Part model, mm, in its own coordinate system. A direction names the side the tool comes from. Round coordinates to 2 decimals unless told otherwise and drop trailing zeros. Write each loop counter-clockwise with the first axis right and the second up, starting at its lowest first coordinate (ties: lowest second). Pieces come first, ordered by that corner, then holes. Notation, with made-up numbers: (-38.75, 86) -> (8.25, 86) arc R20 cw to (8.25, 115) -> close; hole circle Ø10 at (55.5, 48). An arc over 180 degrees is marked (long way). Return JSON: item names as keys, results as strings. Group by question number.
(1) Saw through at A-A (y = 6.25). List the corners of the cut face in (x, z).
(2) Mould opens along Z. For faces 3 (the flat face through (0, 12, 0)), 4 (the flat face through (0, 9.8, 0)), 5 (the cylindrical face through (0.66, 9.931, -14.985)), 6 (the cylindrical face through (-2.88, 5.59, 0.64)) say: +Z half, -Z half, draft (parallel to the pull), parting line (faces both ways), or undercut.
(3) Tool access for faces 1 (the cylindrical face through (0.66, 8.246, -14.985)), 2 (the cylindrical face through (-4.43, 8.75, 14.07)): list every direction of +Z, -Z, +X, -X, +Y, -Y with a clear straight run to the whole face (end or side of a thin tool).
(4) Drill centre lines: L1, parallel to X at y = 6.5, z = 0; L2, parallel to Y at x = -1.25, z = -0.5; L3, parallel to X at y = 5, z = 1.5. Where is each one in solid material? Low to high. Write a range as from..to.
(5) Drop flat-ended pins along their axis: pin 1 Ø1.5 at (y, z) = (9, -6.5) entering from -X; pin 2 Ø3 at (y, z) = (7.5, -2) entering from +X; pin 3 Ø1 at (x, z) = (7, 11) entering from +Y. Give the stop position or say it passes through.
from build123d import *

# Parameters (mm, degrees)
SKETCH1_R               = 15
BOSS_EXTRUDE1_DEPTH     = 12
SKETCH2_R               = 2.95
CUT_EXTRUDE1_DEPTH      = 9.8
SKETCH3_W               = 0.578198398
SKETCH3_H               = 0.5
CHAMFER1_SIZE           = 0.5
FILLET1_R               = 35
CHAMFER3_SIZE           = 0.611779298
CUT_EXTRUDE2_DEPTH      = 25.372115214
CUT_EXTRUDE2_DEPTH_BACK = 25.372115214
SKETCH5_W               = 30
SKETCH5_H               = 1.5
CHAMFER4_SIZE           = 0.5


with BuildPart() as part:
    # Sketch1 → Boss-Extrude1 (new body)
    with BuildSketch(Plane(origin=(0, 0, 0), x_dir=(1, 0, 0), z_dir=(0, 1, 0))):
        with Locations(Location((0, 0, 0), (0, 0, 270))):
            Circle(SKETCH1_R)
    extrude(amount=BOSS_EXTRUDE1_DEPTH)

    # Sketch2 → Cut-Extrude1 (cut)
    with BuildSketch(Plane.XZ):
        with Locations(Location((0, 0, 0), (0, 0, 270))):
            Circle(SKETCH2_R)
    extrude(amount=-CUT_EXTRUDE1_DEPTH, mode=Mode.SUBTRACT)

    # Sketch3 → Cut-Revolve1 (revolve, cut)
    with BuildSketch(Plane.XY, mode=Mode.PRIVATE) as cut_revolve1_sk:
        with Locations((15.039099199, 8.75)):
            Rectangle(SKETCH3_W, SKETCH3_H)
        with Locations((15.039099199, 7.75)):
            Rectangle(SKETCH3_W, SKETCH3_H)
    revolve(cut_revolve1_sk.sketch.rotate(Axis((0, 13.00080105, 0), (0, -1, 0)), 90), axis=Axis((0, 13.00080105, 0), (0, -1, 0)), mode=Mode.SUBTRACT)

    # Chamfer1
    chamfer1_edges = [part.edges().sort_by_distance(p)[0] for p in [
        (0, 12, -15),
    ]]
    chamfer(chamfer1_edges, length=CHAMFER1_SIZE)

    # Fillet1
    # the kernel refuses this fillet: 35 mm, written as the material it takes off along each edge
    with BuildSketch(Plane(origin=(0, 12, 0), x_dir=(0, 0, 1), z_dir=(-1, 0, 0))) as fillet1_piece_1:
        with BuildLine():
            CenterArc((9.105086939, -35), FILLET1_R, 80.303678946, 9.696321054)
            Line((9.105086939, 0), (9.105086939, 0.7))
            Line((9.105086939, 0.7), (14.5, 0.7))
            Line((14.5, 0.7), (14.994974747, 0.494974747))
            ThreePointArc((14.994974747, 0.494974747), (15.244974747, 0.244974747), (15.117898261, 0.19))
            Line((15.117898261, 0.19), (15, -0.5))
        make_face()
    revolve(axis=Axis((0, 12, 0), (0, 1, 0)), mode=Mode.SUBTRACT)

    # Chamfer3
    # the kernel refuses this chamfer: 0.611779298, 0.5 mm, written as the material it takes off along each edge
    with BuildSketch(Plane(origin=(0, 11.5, 0), x_dir=(0, 0, 1), z_dir=(-1, 0, 0))) as chamfer3_piece_1:
        with BuildLine():
            Line((15, -CHAMFER3_SIZE), (14.510020918, 0.080148766))
            ThreePointArc((14.510020918, 0.080148766), (14.746676693, 0.042328599), (15, 0))
            Line((15, 0), (15, -CHAMFER3_SIZE))
        make_face()
    revolve(axis=Axis((0, 11.5, 0), (0, 1, 0)), mode=Mode.SUBTRACT)

    # Sketch5 → Cut-Extrude2 (cut, two sides: drawn at the far end of the back side and taken through both)
    with BuildSketch(Plane.XY.offset(-CUT_EXTRUDE2_DEPTH_BACK)):
        with Locations((0, 0.75)):
            Rectangle(SKETCH5_W, SKETCH5_H)
    extrude(amount=CUT_EXTRUDE2_DEPTH + CUT_EXTRUDE2_DEPTH_BACK, mode=Mode.SUBTRACT)

    # Chamfer4
    chamfer4_edges = [part.edges().sort_by_distance(p)[0] for p in [
        (0, 1.5, -15),
    ]]
    chamfer(chamfer4_edges, length=CHAMFER4_SIZE)


solid = part.part
Computed values:
{
 "1": {"outline": "circle Ø30 at (0, 0); hole circle Ø5.9 at (0, 0)"},
 "2": {"face 3": "draft", "face 4": "undercut", "face 5": "parting line", "face 6": "undercut"},
 "3": {"face 1": "+Y, -Y", "face 2": "none"},
 "4": {"L1": "-15..-2.95, 2.95..15", "L2": "9.8..12", "L3": "-14.92..-2.54, 2.54..14.92"},
 "5": {"pin 1": "x = -13.85", "pin 2": "x = 14.99", "pin 3": "y = 11.83"}
}
